Geometry check sheet. Reference: the model listing, model coordinates, mm. A direction names the side the tool comes from. Round coordinates to 2 decimals unless told otherwise and drop trailing zeros. Loops run counter-clockwise (first coordinate to the right, second up) from the corner with the lowest first, then second, coordinate; pieces in that order, holes last.
```python
from build123d import *

# Parameters (mm, degrees)
BOSS_EXTRUDE1_DEPTH = 13.2842
SKETCH2_R           = 5.588
BOSS_EXTRUDE2_DEPTH = 1.4986
BOSS_EXTRUDE3_DEPTH = 114.04854
CHAMFER1_SIZE       = 0.508
CHAMFER2_SIZE       = 0.254


with BuildPart() as part:
    # Sketch1 → Boss-Extrude1 (new body)
    with BuildSketch(Plane.XZ.offset(25.4)):
        Polygon((-45.639482135, -16.669011646), (-41.973307925, -23.019011646), (-34.640959507, -23.019011646), (-30.974785297, -16.669011646), (-34.640959507, -10.319011646), (-41.973307925, -10.319011646), align=None)
    extrude(amount=-BOSS_EXTRUDE1_DEPTH)

    # Sketch2 → Boss-Extrude2 (add)
    with BuildSketch(Plane(origin=(0, -12.1158, 0), x_dir=(-1, 0, 0), z_dir=(0, 1, 0))):
        with Locations((38.307133716, -16.669011646)):
            Circle(SKETCH2_R)
    extrude(amount=BOSS_EXTRUDE2_DEPTH)

    # Sketch3 → Boss-Extrude3 (add)
    with BuildSketch(Plane.XZ.offset(10.6172)):
        Polygon((-45.639482135, -16.669011646), (-41.973307925, -23.019011646), (-34.640959507, -23.019011646), (-30.974785297, -16.669011646), (-34.640959507, -10.319011646), (-41.973307925, -10.319011646), align=None)
    extrude(amount=-BOSS_EXTRUDE3_DEPTH)

    # Sketch4 → Revolve1 (revolve)
    with BuildSketch(Plane(origin=(0, 0, -16.669011646), x_dir=(-1, 0, 0), z_dir=(0, 0, -1))):
        Polygon((35.144833716, -45.212), (38.307133716, -45.212), (38.307133716, -25.4), (33.557333716, -25.4), (33.557333716, -32.512), (35.144833716, -32.512), align=None)
    revolve(axis=Axis((-38.307133716, -45.212, -16.669011646), (0, 1, 0)))

    # Chamfer1
    chamfer1_edges = [part.edges().sort_by_distance(p)[0] for p in [
        (-41.469433716, -45.212, -16.669011646),
        (-43.056933716, -32.512, -16.669011646),
    ]]
    chamfer(chamfer1_edges, length=CHAMFER1_SIZE)

    # Chamfer2
    chamfer2_edges = [part.edges().sort_by_distance(p)[0] for p in [
        (-43.80639503, 103.43134, -13.494011646),
        (-38.307133716, 103.43134, -10.319011646),
        (-32.807872402, 103.43134, -13.494011646),
        (-32.807872402, 103.43134, -19.844011646),
        (-38.307133716, 103.43134, -23.019011646),
        (-43.80639503, 103.43134, -19.844011646),
    ]]
    chamfer(chamfer2_edges, length=CHAMFER2_SIZE)


solid = part.part
```
1) Gauge pin test, flat ends, axial feed: pin 1 (4 mm diameter, centred on y = -12.5, z = -13, fed in from -X); pin 2 (8 mm diameter, centred on x = -44, y = -25, fed in from +Z); pin 3 (2 mm diameter, centred on x = -43, y = 20, fed in from -Z). Record the tip position at first contact, or that the pin passes through.
Report:
pin 1: stops at x = -44.68
pin 2: stops at z = -10.32
pin 3: stops at z = -22.97
2) Sectioned sample at A-A, the plane y = 9. Record the cut outline in (x, z).
Report:
outline: (-45.64, -16.67) - (-41.97, -23.02) - (-34.64, -23.02) - (-30.97, -16.67) - (-34.64, -10.32) - (-41.97, -10.32) - close
3) Scan lines: line 1 along Y through (x, z) = (-42.75, -12.75); line 2 along Y through (x, z) = (-36, -19.5); line 3 along Z through (x, y) = (-38.25, -33.5). Record each from-to range of solid material in increasing order.
Report:
line 1: y = -25.4 to -12.12, -10.62 to 103.43
line 2: y = -32.51 to 103.43
line 3: z = -19.83 to -13.51
4) Access from +Z, -Z, +X, -X, +Y, -Y to the whole of each face (thin tool, end or side, straight path). Record for faces 1 (the face through (-33, -10.617, -14)), 2 (the face through (-43.78, -18.85, -13.45)), 3 (the face through (-39.337, -28.748, -12.032)).
Report:
face 1: none
face 2: +Z, -X, +Y, -Y
face 3: -Y
5) Sectioned sample at B-B, the plane y = -28.5. Record the cut outline in (x, z).
Report:
outline: circle Ø9.5 at (-38.31, -16.67)
